Drawing for the job (mm, zero at the part's lowest x, y, z). Give positions to 0.01 mm unless a question says otherwise; leave off trailing zeros. Write each loop counter-clockwise with the first axis right and the second up, starting at its lowest first coordinate (ties: lowest second). Pieces come first, ordered by that corner, then holes. Notation, with made-up numbers: (-9.75, 41) - (-2.75, 41) arc R21 ccw to (-2.75, 74) - close; hole circle Ø8 at (11, 85.5). An arc over 180 degrees is marked (long way). Use CSV: the item, a comma, the result in double quotes.
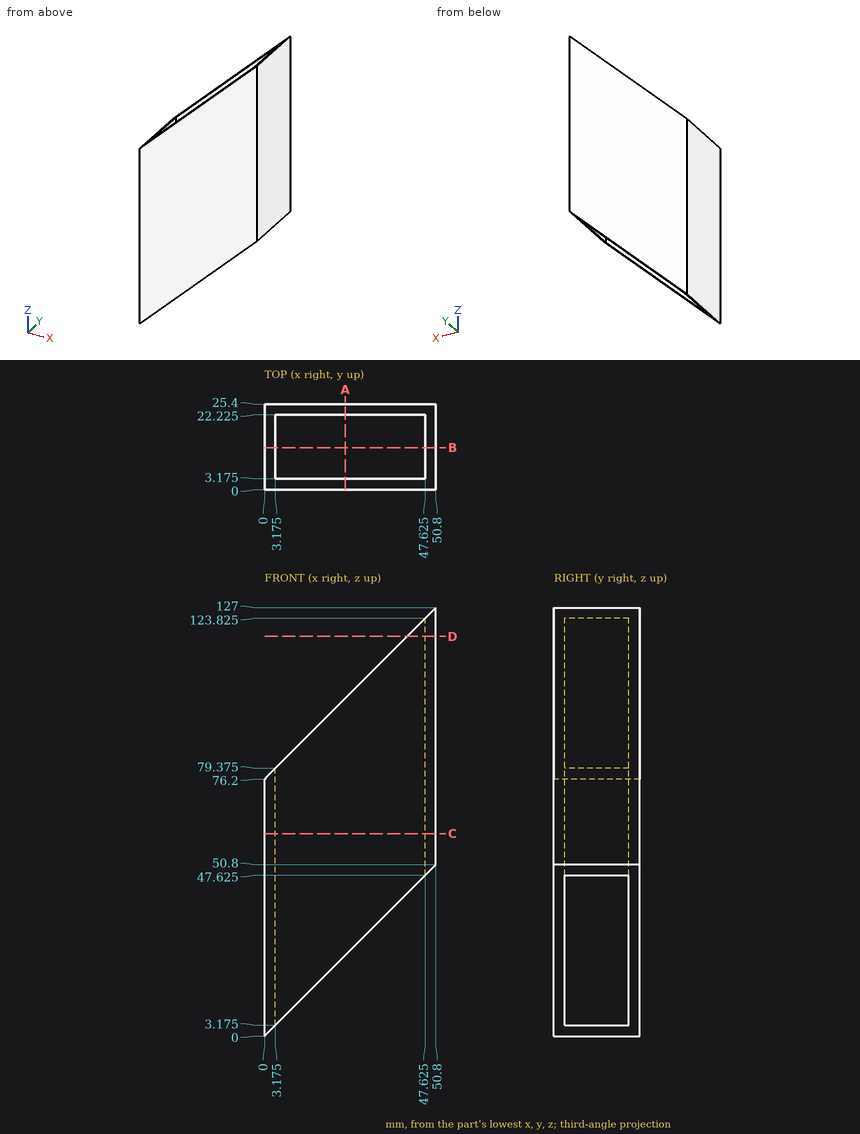
(1) Saw through at C-C, the plane z = 60. List the corners of the cut face in (x, y) (3 decimals), then the cut area to 3 significant figures.
Checked values:
outline,"(0, 0) - (50.8, 0) - (50.8, 25.4) - (0, 25.4) - close; hole (3.175, 3.175) - (47.625, 3.175) - (47.625, 22.225) - (3.175, 22.225) - close"
area,"444 mm^2"
(2) Saw through at A-A, the plane x = 24. List the corners of the cut face in (y, z) (3 decimals), then the cut area to 3 significant figures.
Checked values:
outline,"(0, 24) - (3.175, 24) - (3.175, 100.2) - (0, 100.2) - close; (22.225, 24) - (25.4, 24) - (25.4, 100.2) - (22.225, 100.2) - close"
area,"484 mm^2"
(3) Wall check: probe 1 along Y at (x, z) = (9, 34) (3 decimals); probe 2 along X at (y, z) = (20, 61.5) (3 decimals); probe 3 along X at (y, z) = (5.5, 13) (3 decimals). Give the ranges that are in metal, low to high. Write a range as [from, to].
Checked values:
probe 1,"y = [0, 3.175], [22.225, 25.4]"
probe 2,"x = [0, 3.175], [47.625, 50.8]"
probe 3,"x = [0, 3.175]"
(4) Flat gauge pins, fed straight in: P1, Ø5, axis at x = 45, y = 22, coming from the -Z side; P2, Ø9.5, axis at y = 14.5, z = 103, coming from the -X side (3 decimals); P3, Ø9.5, axis at y = 9.5, z = 33.5, coming from the +X side (3 decimals); P4, Ø4, axis at x = 8.5, y = 19, coming from the +Z side. Where does each tip first touch, or does it go through?
Checked values:
P1,"stops at z = 42.51"
P2,"stops at x = 47.625"
P3,"stops at x = 3.175"
P4,"passes through"
(5) Saw through at B-B, the plane y = 12.5. List the corners of the cut face in (x, z) (3 decimals), then the cut area to 3 significant figures.
Checked values:
outline,"(0, 0) - (3.175, 3.175) - (3.175, 79.375) - (0, 76.2) - close; (47.625, 47.625) - (50.8, 50.8) - (50.8, 127) - (47.625, 123.825) - close"
area,"484 mm^2"
(6) Saw through at D-D, the plane z = 118.5. List the corners of the cut face in (x, y) (3 decimals), then the cut area to 3 significant figures.
Checked values:
outline,"(42.3, 0) - (50.8, 0) - (50.8, 25.4) - (42.3, 25.4) - (42.3, 22.225) - (47.625, 22.225) - (47.625, 3.175) - (42.3, 3.175) - close"
area,"114 mm^2"
